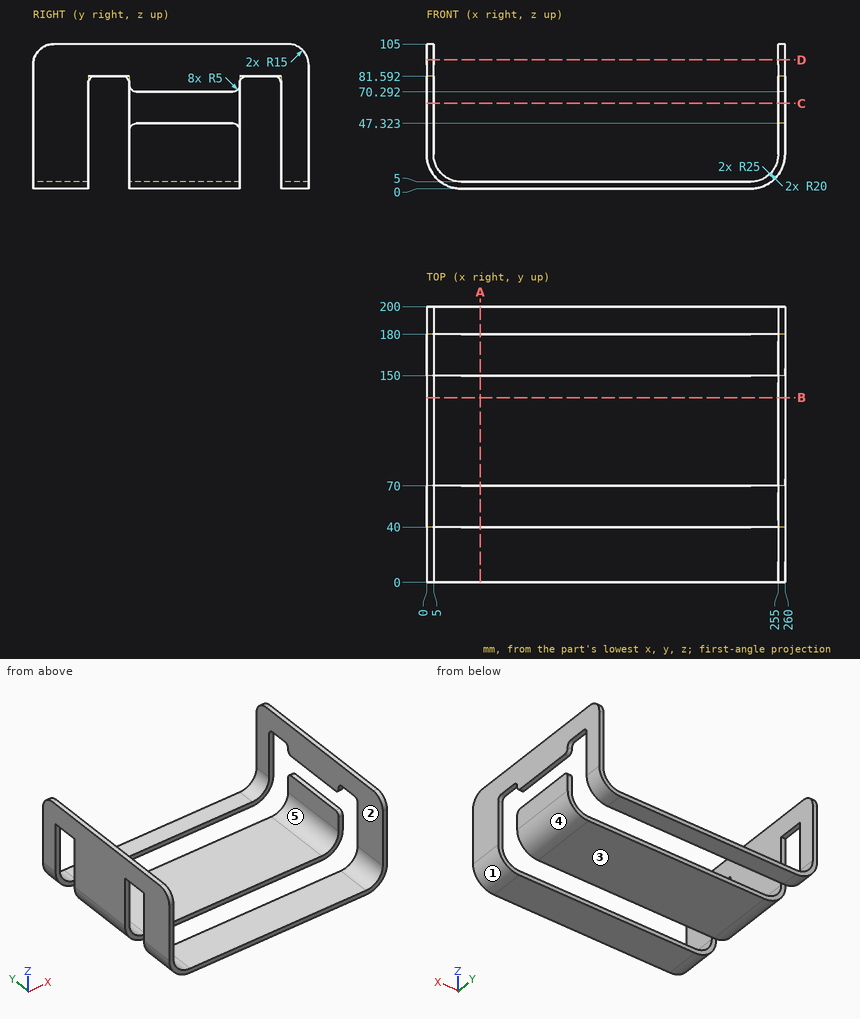
Design review of the part shown in the three views and the two pictorial views. Dimensions are in mm from the part's minimum x, y and z. A direction names the side the tool comes from. Round coordinates to 2 decimals unless told otherwise and drop trailing zeros. Loops run counter-clockwise (first coordinate to the right, second up) from the corner with the lowest first, then second, coordinate; pieces in that order, holes last.
(1) We need section B-B (y = 134). Give the boundary of the cut face in (x, z), plus the area to 3 significant figures.
Returned:
outline: (0, 25) arc R25 ccw to (25, 0) - (235, 0) arc R25 ccw to (260, 25) - (260, 47.32) - (255, 47.32) - (255, 25) arc R20 cw to (235, 5) - (25, 5) arc R20 cw to (5, 25) - (5, 105) - (0, 105) - close; (255, 70.29) - (260, 70.29) - (260, 105) - (255, 105) - close
area: 2,090 mm2
(2) Wall thickness on line 1 along X through (y, z) = (16.5, 46.5); line 2 along Z through (x, y) = (86.5, 94.5): over which ranges is each line inside the solid? List them lowest first.
Returned:
line 1: x = 0 to 5, 255 to 260
line 2: z = 0 to 5
(3) We need section D-D (z = 93.5). Give the boundary of the cut face in (x, y), plus the area to 3 significant figures.
Returned:
outline: (0, 0.41) - (5, 0.41) - (5, 199.59) - (0, 199.59) - close; (255, 0.41) - (260, 0.41) - (260, 199.59) - (255, 199.59) - close
area: 1,990 mm2
(4) Mouldability with a two-part tool opening along X and no side actions: class the marked faces 3, 4 and 5 as released by +X, released by -X, zero draft, split by the parting line, or undercut.
Returned:
face 3: zero draft
face 4: released by +X
face 5: undercut
(5) We need section A-A (x = 39). Give the boundary of the cut face in (y, z).
Returned:
outline: (0, 0) - (40, 0) - (40, 5) - (0, 5) - close; (70, 0) - (150, 0) - (150, 5) - (70, 5) - close; (180, 0) - (200, 0) - (200, 5) - (180, 5) - close
(6) Clearance check with flat-ended pins moving along their axes: P1, Ø2, axis at y = 88.5, z = 64.5, coming from the +X side; P2, Ø2.5, axis at x = 258, y = 116.5, coming from the -Z side (1 decimal); P3, Ø4, axis at x = 100, y = 131, coming from the -Z side; P4, Ø12, axis at x = 176.5, y = 20.5, coming from the +Z side. State where each tip first meets the part, or that it passes through.
Returned:
P1: stops at x = 5
P2: stops at z = 12.7
P3: stops at z = 0
P4: stops at z = 5
(7) Tool access review of the marked faces 1 and 2: name each direction out of +Z, -Z, +X, -X, +Y, -Y from which nothing blocks a thin tool from reaching the whole face with its end or side.
Returned:
face 1: -Z, +X, +Y, -Y
face 2: +Z, +Y, -Y
(8) We need section C-C (z = 62). Give the boundary of the cut face in (x, y), plus the area to 3 significant figures.
Returned:
outline: (0, 0) - (5, 0) - (5, 40) - (0, 40) - close; (0, 70) - (5, 70) - (5, 150) - (0, 150) - close; (0, 180) - (5, 180) - (5, 200) - (0, 200) - close; (255, 0) - (260, 0) - (260, 40) - (255, 40) - close; (255, 180) - (260, 180) - (260, 200) - (255, 200) - close
area: 1,000 mm2
